```python
from build123d import *

# Parameters (mm, degrees)
SKETCH2_W           = 63.246
SKETCH2_H           = 39.058596
BOSS_EXTRUDE1_DEPTH = 4.800000052
SKETCH5_W           = 4.800000052
SKETCH5_H           = 7.8117192
CUT_EXTRUDE1_DEPTH  = 75.489398158
SKETCH6_R           = 1.750000056
CUT_EXTRUDE2_DEPTH  = 75.489398158


with BuildPart() as part:
    # Sketch2 → Boss-Extrude1 (new body)
    with BuildSketch(Plane.XY):
        with Locations((31.623, 19.529298)):
            Rectangle(SKETCH2_W, SKETCH2_H)
    extrude(amount=BOSS_EXTRUDE1_DEPTH)

    # Sketch5 → Cut-Extrude1 (cut, through all)
    with BuildSketch(Plane.XY.offset(4.800000052)):
        with Locations((60.845999974, 11.7175788)):
            Rectangle(SKETCH5_W, SKETCH5_H)
        with Locations((60.845999974, 27.3410172)):
            Rectangle(SKETCH5_W, SKETCH5_H)
    extrude(amount=-CUT_EXTRUDE1_DEPTH, mode=Mode.SUBTRACT)

    # Sketch6 → Cut-Extrude2 (cut, through all)
    with BuildSketch(Plane.XY.offset(4.800000052)):
        with Locations((39.032113706, 19.529298)):
            Circle(SKETCH6_R)
    extrude(amount=-CUT_EXTRUDE2_DEPTH, mode=Mode.SUBTRACT)


solid = part.part
```
Here's how the part is built. I have some questions about the finished solid (model axes, mm). A direction names the side the tool comes from. Coordinates: 2 decimals unless noted, no trailing zeros. Write each loop counter-clockwise with the first axis right and the second up, starting at its lowest first coordinate (ties: lowest second). Pieces come first, ordered by that corner, then holes. Notation, with made-up numbers: (72, 36) -> (119, 36) arc R9 ccw to (119, 40) -> close; hole circle Ø3 at (0.25, 46). An arc over 180 degrees is marked (long way). Use a Markdown table: item, result. Add a question column.
(1) We'd pull the mould along Y, two halves only. Please class faces 3 (the flat face through (63.246, 35, 2)), 4 (the flat face through (31, 39.059, 2)), 5 (the cylindrical face through (37.284, 19.606, 2.434)): +Y half, -Y half, draft (parallel to the pull), parting line (faces both ways), or undercut.
(2) If we section it at A-A, the plane z = 1.3: Write out the boundary of the cut face in (x, y), and give its area (3 significant figures).
(3) For faces 1 (the flat face through (31, 20, 0)), 2 (the flat face through (61, 7.812, 2)), which set-ups out of +Z, -Z, +X, -X, +Y, -Y let a thin tool reach every point of the face, with its end or its side?
(4) Please list where these lines run through material, in increasing order: line 1 (X direction, y = 15.5, z = 4.4); line 2 (X direction, y = 20, z = 1.4); line 3 (X direction, y = 21, z = 1.9).
(5) I'm going to push flat-ended pins straight in: P1, Ø1.5, axis at y = 14, z = 2.5, coming from the -X side; P2, Ø2.5, axis at y = 13, z = 3, coming from the +X side. Where does each tip first touch, or does it pass through?
(6) If we section it at B-B, the plane y = 13: Write out the boundary of the cut face in (x, z), and give its area (3 significant figures).
Outcome:
| question | item | result |
|---|---|---|
| 1 | face 3 | draft |
| 1 | face 4 | +Y half |
| 1 | face 5 | undercut |
| 2 | outline | (0, 0) -> (63.25, 0) -> (63.25, 7.81) -> (58.45, 7.81) -> (58.45, 15.62) -> (63.25, 15.62) -> (63.25, 23.44) -> (58.45, 23.44) -> (58.45, 31.25) -> (63.25, 31.25) -> (63.25, 39.06) -> (0, 39.06) -> close; hole circle Ø3.5 at (39.03, 19.53) |
| 2 | area | 2,390 mm^2 |
| 3 | face 1 | -Z, +X, -X, +Y, -Y |
| 3 | face 2 | +Z, -Z, +X |
| 4 | line 1 | x = 0 to 58.45 |
| 4 | line 2 | x = 0 to 37.35, 40.72 to 63.25 |
| 4 | line 3 | x = 0 to 38.08, 39.98 to 63.25 |
| 5 | P1 | stops at x = 0 |
| 5 | P2 | stops at x = 58.45 |
| 6 | outline | (0, 0) -> (58.45, 0) -> (58.45, 4.8) -> (0, 4.8) -> close |
| 6 | area | 281 mm^2 |
